Input: part model. Units: mm. Frame: model coordinates. A direction names the side the tool comes from. Coordinates: 2 decimals unless noted, no trailing zeros. Write each loop counter-clockwise with the first axis right and the second up, starting at its lowest first coordinate (ties: lowest second). Pieces come first, ordered by that corner, then holes. Notation, with made-up numbers: (1, 28) - (52, 28) arc R25 cw to (52, 40) - close; hole circle Ø4 at (-20, 49). An arc over 180 degrees is marked (long way). Use a Markdown table: item, result. Add a question column.
Q1. Material intervals for probe 1 along X at (y, z) = (2.25, 0); probe 2 along Z at (x, y) = (-9.5, 0); probe 3 along Y at (x, z) = (-13.5, 0), sorted ascending. Write a range as from..to.
Q2. Section query B-B (x = 19). Return the cut outline in (y, z), then the cut area to 3 significant figures.
Q3. Mould query, pull axis Y, two halves, no side actions, for faces 1 (the face through (-0.74, -9.76, -2.17)), 2 (the face through (-9.395, 5.525, -3.131)), 3 (the face through (-10.713, 0.631, -2.003)), 4 (the face through (-3.56, 0.11, 0.35)). Classes: released by +Y, released by -Y, zero draft, split by the parting line, or undercut.
Q4. Pin query (flat end, axial travel): P1, Ø2, axis at x = -11.5, y = 0.5, coming from the -Z side; P2, Ø1.5, axis at x = 49, z = 0.5, coming from the +Y side; P3, Ø5, axis at x = 32, z = 2.5, coming from the -Y side. Return the tip coordinate at first contact, or that it passes through.
Q5. Set-up query: faces 5 (the face through (-9.395, -5.525, 3.131)), 6 (the face through (-9, 0, 6.35)), 7 (the face through (-9.395, -5.474, -3.219)), 8 (the face through (-9, 0, -6.35)). Return all of +Z, -Z, +X, -X, +Y, -Y with unobstructed straight access to the full face (end or side cutting, diameter ignored); none if empty.
Q6. Section query C-C (x = 62.7). Return the cut outline in (y, z).
Q7. Section query A-A (x = -10). Return the cut outline in (y, z), then the cut area to 3 significant figures.
from build123d import *

# Parameters (mm, degrees)
SKETCH_1_R               = 7.9
EXTRUDE_1_DEPTH          = 75
SKETCH_3_R               = 10
EXTRUDE_2_DEPTH          = 2
EXTRUDE_3_DEPTH          = 15
CHAMFER_1_SIZE           = 0.5
M5X0_8_1_D               = 4.2
M5X0_8_1_DEPTH           = 12.4
M5X0_8_1_TIP             = 1.2618073
SKETCH_5_R               = 3.1
CUT_EXTRUDE_1_DEPTH      = 11
CUT_EXTRUDE_1_DEPTH_BACK = 11
CHAMFER_2_SIZE           = 1


with BuildPart() as part:
    # 草图1 → 凸台-拉伸1 (new body)
    with BuildSketch(Plane(origin=(0, 0, 0), x_dir=(0, 0, -1), z_dir=(1, 0, 0))):
        Circle(SKETCH_1_R)
    extrude(amount=EXTRUDE_1_DEPTH)

    # 草图3 → 凸台-拉伸2 (add)
    with BuildSketch(Plane.ZY):
        Circle(SKETCH_3_R)
    extrude(amount=EXTRUDE_2_DEPTH)

    # 草图4 → 凸台-拉伸3 (add)
    with BuildSketch(Plane.ZY.offset(2)):
        Polygon((6.35, 3.666174209), (0, 7.332348419), (-6.35, 3.666174209), (-6.35, -3.666174209), (0, -7.332348419), (6.35, -3.666174209), align=None)
    extrude(amount=EXTRUDE_3_DEPTH)

    # 倒角1
    chamfer_1_edges = [part.edges().sort_by_distance(p)[0] for p in [
        (-2, 0, -10),
    ]]
    chamfer(chamfer_1_edges, length=CHAMFER_1_SIZE)

    # M5x0.8 螺纹孔1
    with Locations(Plane.ZY.offset(17)):
        with Locations((0, 0)):
            Hole(M5X0_8_1_D / 2, depth=M5X0_8_1_DEPTH)
            with Locations((0, 0, -(M5X0_8_1_DEPTH + M5X0_8_1_TIP / 2))):  # 118° drill point
                Cone(0, M5X0_8_1_D / 2, M5X0_8_1_TIP, mode=Mode.SUBTRACT)

    # 草图5 → 切除-拉伸1 (cut, two sides)
    with BuildSketch(Plane(origin=(0, 0, 0), x_dir=(1, 0, 0), z_dir=(0, 1, 0))) as cut_extrude_1_sk:
        with Locations((62.7, 0)):
            Circle(SKETCH_5_R)
    extrude(amount=CUT_EXTRUDE_1_DEPTH, mode=Mode.SUBTRACT)
    extrude(cut_extrude_1_sk.sketch, amount=-CUT_EXTRUDE_1_DEPTH_BACK, mode=Mode.SUBTRACT)

    # 倒角2
    chamfer_2_edges = [part.edges().sort_by_distance(p)[0] for p in [
        (75, 0, 7.9),
    ]]
    chamfer(chamfer_2_edges, length=CHAMFER_2_SIZE)


solid = part.part
Values follow:
| question | item | result |
|---|---|---|
| 1 | probe 1 | -17..59.6, 65.8..75 |
| 1 | probe 2 | -6.35..-2.1, 2.1..6.35 |
| 1 | probe 3 | -7.33..-2.1, 2.1..7.33 |
| 2 | outline | circle Ø15.8 at (0, 0) |
| 2 | area | 196 mm2 |
| 3 | face 1 | split by the parting line |
| 3 | face 2 | released by +Y |
| 3 | face 3 | undercut |
| 3 | face 4 | undercut |
| 4 | P1 | z = -6.35 |
| 4 | P2 | y = 7.9 |
| 4 | P3 | y = -7.9 |
| 5 | face 5 | +Z, -X, -Y |
| 5 | face 6 | +Z, -X, +Y, -Y |
| 5 | face 7 | -Z, -X, -Y |
| 5 | face 8 | -Z, -X, +Y, -Y |
| 6 | outline | (-7.27, -3.1) arc R7.9 ccw to (7.27, -3.1) - close; (-7.27, 3.1) - (7.27, 3.1) arc R7.9 ccw to start |
| 7 | outline | (-7.33, 0) - (-3.67, -6.35) - (3.67, -6.35) - (7.33, 0) - (3.67, 6.35) - (-3.67, 6.35) - close; hole circle Ø4.2 at (0, 0) |
| 7 | area | 126 mm2 |
